Model file for the job. Use its own axes, mm. A direction names the side the tool comes from. Coordinates: 2 decimals unless noted, no trailing zeros. Order: outer loops, then holes, each group sorted by start corner. A loop starts at its lowest first (then second) coordinate and runs counter-clockwise, first axis right, second up. Notation, with made-up numbers: (4, 72.25) -> (18, 72.25) arc R27 cw to (18, 100.25) -> close; hole circle Ø10 at (2.25, 76.5). An arc over 180 degrees is marked (long way). Return JSON: item names as keys, results as strings. Group by question number.
1) Pull direction X, two halves, no side cores. Call faces 3 (the flat face through (39, 17, 8)), 4 (the cylindrical face through (36.786, 7.536, 3.944)): +X half, -X half, draft (parallel to the pull), parting line (faces both ways), or undercut.
2) Cut at C-C (x = 13.5). Write the cut outline in (y, z), and give its area (3 significant figures).
3) Flat gauge pins, fed straight in: pin 1 (5 mm diameter, centred on x = 73, y = 8, fed in from -Z); pin 2 (1.6 mm diameter, centred on x = 36, z = 3.5, fed in from +Y); pin 3 (1.4 mm diameter, centred on x = 45, y = 33, fed in from -Z). Where does each tip first touch, or does it go through?
4) Probe line 1 (Y direction, x = 23, z = 7.45); line 2 (Y direction, x = 60, z = 4); line 3 (X direction, y = 13, z = 2). List the from-to ranges inside material, lowest first.
5) Cut at D-D (z = 3.5). State how many separate pieces and enclosed holes the cut face has, and give its area (3 significant figures).
6) Which spindle directions (+Z, -Z, +X, -X, +Y, -Y) get a long thin tool onto all of the face, cutting with end or side? Do faces 1 (the flat face through (20.921, 11.534, 2.958)), 2 (the cylindrical face through (33.478, 10.466, 6.274)). Say none if no direction does.
7) Cut at B-B (x = 73). Write the cut outline in (y, z), and give its area (3 significant figures).
8) Cut at A-A (y = 25). Write the cut outline in (x, z).
from build123d import *

# Parameters (mm, degrees)
SKETCH_2_W           = 80
SKETCH_2_H           = 34
SKETCH_2_R           = 4.05
EXTRUDE_1_DEPTH      = 8
SKETCH_3_R           = 2.55
CUT_EXTRUDE_1_DEPTH  = 88.292611371
CUT_EXTRUDE_2_DEPTH  = 88.292611371
SKETCH_5_R           = 1.55
CUT_EXTRUDE_3_DEPTH  = 88.292611371
CUT_EXTRUDE_5_DEPTH  = 4.5
SKETCH_11_R          = 1.55
CUT_EXTRUDE_7_DEPTH  = 88.292611371
CUT_EXTRUDE_11_DEPTH = 2
CUT_EXTRUDE_13_DEPTH = 6


with BuildPart() as part:
    # 草图2 → 凸台-拉伸1 (new body)
    with BuildSketch(Plane.XY):
        with Locations((40, 17)):
            Rectangle(SKETCH_2_W, SKETCH_2_H)
        with Locations((7, 8)):
            Circle(SKETCH_2_R, mode=Mode.SUBTRACT)
        with Locations((40, 10)):
            Circle(SKETCH_2_R, mode=Mode.SUBTRACT)
        with Locations((73, 8)):
            Circle(SKETCH_2_R, mode=Mode.SUBTRACT)
    extrude(amount=EXTRUDE_1_DEPTH)

    # 草图3 → 切除-拉伸1 (cut, through all)
    with BuildSketch(Plane.XY.offset(8)):
        with Locations((23, 8)):
            Circle(SKETCH_3_R)
        with Locations((57, 8)):
            Circle(SKETCH_3_R)
    extrude(amount=-CUT_EXTRUDE_1_DEPTH, mode=Mode.SUBTRACT)

    # 草图4 → 切除-拉伸2 (cut, through all)
    with BuildSketch(Plane(origin=(80, 0, 0), x_dir=(0, 0, -1), z_dir=(1, 0, 0))):
        Polygon((-1.5, 32.2), (-2.5, 32.2), (-2.5, 34), (0, 34), (0, 28.8), (-1.5, 28.8), align=None)
    extrude(amount=-CUT_EXTRUDE_2_DEPTH, mode=Mode.SUBTRACT)

    # 草图5 → 切除-拉伸3 (cut, through all)
    with BuildSketch(Plane.XY.offset(8)):
        with Locations((48, 10)):
            Circle(SKETCH_5_R)
        with Locations((32, 10)):
            Circle(SKETCH_5_R)
    extrude(amount=-CUT_EXTRUDE_3_DEPTH, mode=Mode.SUBTRACT)

    # 草图8 → 切除-拉伸5 (cut)
    with BuildSketch(Plane(origin=(0, 0, 0), x_dir=(-1, 0, 0), z_dir=(0, 0, -1))):
        Polygon((-45.15, 8.354551733), (-45.15, 11.645448267), (-48, 13.290896534), (-50.85, 11.645448267), (-50.85, 8.354551733), (-48, 6.709103466), align=None)
        Polygon((-29.15, 8.354551733), (-29.15, 11.645448267), (-32, 13.290896534), (-34.85, 11.645448267), (-34.85, 8.354551733), (-32, 6.709103466), align=None)
    extrude(amount=-CUT_EXTRUDE_5_DEPTH, mode=Mode.SUBTRACT)

    # 草图11 → 切除-拉伸7 (cut, through all)
    with BuildSketch(Plane(origin=(0, 0, 0), x_dir=(-1, 0, 0), z_dir=(0, 0, -1))):
        with Locations((-60, 25)):
            Circle(SKETCH_11_R)
        with Locations((-20, 25)):
            Circle(SKETCH_11_R)
    extrude(amount=-CUT_EXTRUDE_7_DEPTH, mode=Mode.SUBTRACT)

    # 草图19 → 切除-拉伸11 (cut)
    with BuildSketch(Plane(origin=(0, 0, 2.5), x_dir=(-1, 0, 0), z_dir=(0, 0, -1))):
        with BuildLine():
            Line((-25, 34), (-55.247938178, 34))
            Line((-55.247938178, 34), (-55.247938178, 33.2))
            ThreePointArc((-55.247938178, 33.2), (-54.747938178, 32.7), (-54.247938178, 33.2))
            Line((-54.247938178, 33.2), (-26, 33.2))
            ThreePointArc((-26, 33.2), (-25.5, 32.7), (-25, 33.2))
            Line((-25, 33.2), (-25, 34))
        make_face()
    extrude(amount=-CUT_EXTRUDE_11_DEPTH, mode=Mode.SUBTRACT)

    # 草图7 → 切除-拉伸13 (cut)
    with BuildSketch(Plane(origin=(0, 0, 0), x_dir=(-1, 0, 0), z_dir=(0, 0, -1))):
        Polygon((-52.9, 5.632863896), (-52.9, 10.367136104), (-57, 12.734272207), (-61.1, 10.367136104), (-61.1, 5.632863896), (-57, 3.265727793), align=None)
        Polygon((-18.9, 5.632863896), (-18.9, 10.367136104), (-23, 12.734272207), (-27.1, 10.367136104), (-27.1, 5.632863896), (-23, 3.265727793), align=None)
    extrude(amount=-CUT_EXTRUDE_13_DEPTH, mode=Mode.SUBTRACT)


solid = part.part
Answers below:
{
 "1": {"face 3": "draft", "face 4": "undercut"},
 "2": {"outline": "(0, 0) -> (28.8, 0) -> (28.8, 1.5) -> (32.2, 1.5) -> (32.2, 2.5) -> (34, 2.5) -> (34, 8) -> (0, 8) -> close", "area": "262 mm^2"},
 "3": {"pin 1": "passes through", "pin 2": "stops at y = 33.2", "pin 3": "stops at z = 2.5"},
 "4": {"line 1": "y = 0 to 5.45, 10.55 to 34", "line 2": "y = 0 to 5, 11 to 23.45, 26.55 to 34", "line 3": "x = 0 to 31.5, 32.5 to 37.28, 42.72 to 47.5, 48.5 to 80"},
 "5": {"separate pieces": "1", "enclosed holes": "9", "area": "2,350 mm^2"},
 "6": {"face 1": "-Z", "face 2": "+Z, -Z"},
 "7": {"outline": "(0, 0) -> (3.95, 0) -> (3.95, 8) -> (0, 8) -> close; (12.05, 0) -> (28.8, 0) -> (28.8, 1.5) -> (32.2, 1.5) -> (32.2, 2.5) -> (34, 2.5) -> (34, 8) -> (12.05, 8) -> close", "area": "198 mm^2"},
 "8": {"outline": "(0, 0) -> (18.45, 0) -> (18.45, 8) -> (0, 8) -> close; (21.55, 0) -> (58.45, 0) -> (58.45, 8) -> (21.55, 8) -> close; (61.55, 0) -> (80, 0) -> (80, 8) -> (61.55, 8) -> close"}
}
